Model file for the job. Use its own axes, mm. A direction names the side the tool comes from. Round coordinates to 2 decimals unless told otherwise and drop trailing zeros. Loops run counter-clockwise (first coordinate to the right, second up) from the corner with the lowest first, then second, coordinate; pieces in that order, holes last. Notation, with made-up numbers: M 9,-35 L 63,-35 A15 ccw 63,-18 Z; hole C 34.25,53.25 d10. An arc over 180 degrees is marked long. Use a Markdown table: item, result. Add a question column.
Item 1: Saw through at D-D on y = 0. Write the cut outline in (x, z), then the cut area to 3 significant figures.
Item 2: Saw through at B-B on x = -11. Write the cut outline in (y, z).
Item 3: Saw through at C-C on z = -5. Write the cut outline in (x, y) (3 decimals).
Item 4: Two-plate mould, pull along X, no slides. Class faces 1 (the cylindrical face through (15.5, -0.11, 4.88)), 2 (the cylindrical face through (-1.73, 0.04, 7.81)), 3 (the flat face through (13, 8, 8)): +X half, -X half, draft (parallel to the pull), parting line (faces both ways), or undercut.
Item 5: Pin check, flat tips, straight feed: P1, Ø2, axis at x = -6.5, y = -4.5, coming from the +Z side; P2, Ø17, axis at x = -7, z = 0, coming from the +Y side; P3, Ø1, axis at x = -8.5, y = 2, coming from the -Z side; P4, Ø2, axis at x = -3.5, z = 8.5, coming from the +Y side. Stop position of each tip, or through.
Item 6: Saw through at A-A on z = 0. Give the number of separate pieces and of enclosed holes in the cut face, then the cut area to 3 significant figures.
Item 7: Tool access for faces 4 (the flat face through (13, 7.5, -10)), 5 (the flat face through (-6, 2.5, -6)), 6 (the cylindrical face through (16.453, -7.753, 5.181)), 7 (the flat face through (6, -2.5, -6)), 8 (the flat face through (-13, -8, 8)): list every direction of +Z, -Z, +X, -X, +Y, -Y with a clear straight run to the whole face (end or side of a thin tool).
Item 8: Wall check: L1, parallel to Y at x = 15.5, z = 7.5; L2, parallel to Z at x = -5.5, y = -1.15; L3, parallel to Z at x = 0, y = -5.9. Give the ranges that are in metal, low to high. Write a range as from..to.
```python
from build123d import *

# Parameters (mm, degrees)
SKETCH2_R          = 1.25
SKETCH2_R_2        = 8
CUT_EXTRUDE1_DEPTH = 10


with BuildPart() as part:
    # Sketch1 → Revolve1 (revolve)
    with BuildSketch(Plane.XY):
        Polygon((15, 8), (17.25, 8), (17.25, 7.5), (16.25, 7.5), (16.25, -7.5), (17.25, -7.5), (17.25, -8), (15, -8), (15, -2.5), (0, -2.5), (0, 2.5), (15, 2.5), align=None)
    revolve(axis=Axis((0, 8.982990787, 0), (0, -1, 0)))

    # Sketch2 → Cut-Extrude1 (cut, symmetric)
    with BuildSketch(Plane(origin=(0, 2.5, 0), x_dir=(1, 0, 0), z_dir=(0, 1, 0))):
        with Locations((11, 0)):
            Circle(SKETCH2_R)
        with Locations((5.5, -9.526279442)):
            Circle(SKETCH2_R)
        with Locations((-5.5, -9.526279442)):
            Circle(SKETCH2_R)
        with Locations((-11, 0)):
            Circle(SKETCH2_R)
        with Locations((-5.5, 9.526279442)):
            Circle(SKETCH2_R)
        with Locations((5.5, 9.526279442)):
            Circle(SKETCH2_R)
        Circle(SKETCH2_R_2)
    extrude(amount=CUT_EXTRUDE1_DEPTH, both=True, mode=Mode.SUBTRACT)


solid = part.part
```
Entries:
| question | item | result |
|---|---|---|
| 1 | outline | C 0,0 d32.5; hole C -11,0 d2.5; hole C 0,0 d16; hole C -5.5,-9.53 d2.5; hole C -5.5,9.53 d2.5; hole C 5.5,-9.53 d2.5; hole C 5.5,9.53 d2.5; hole C 11,0 d2.5 |
| 1 | area | 599 mm2 |
| 2 | outline | M -8,-13.29 L -7.5,-13.29 L -7.5,-11.96 L 7.5,-11.96 L 7.5,-13.29 L 8,-13.29 L 8,-10.2 L 2.5,-10.2 L 2.5,-1.25 L -2.5,-1.25 L -2.5,-10.2 L -8,-10.2 Z; M -8,10.2 L -2.5,10.2 L -2.5,1.25 L 2.5,1.25 L 2.5,10.2 L 8,10.2 L 8,13.29 L 7.5,13.29 L 7.5,11.96 L -7.5,11.96 L -7.5,13.29 L -8,13.29 Z |
| 3 | outline | M -16.509,-8 L -14.142,-8 L -14.142,-2.5 L -6.245,-2.5 L -6.245,2.5 L -14.142,2.5 L -14.142,8 L -16.509,8 L -16.509,7.5 L -15.462,7.5 L -15.462,-7.5 L -16.509,-7.5 Z; M 6.245,-2.5 L 14.142,-2.5 L 14.142,-8 L 16.509,-8 L 16.509,-7.5 L 15.462,-7.5 L 15.462,7.5 L 16.509,7.5 L 16.509,8 L 14.142,8 L 14.142,2.5 L 6.245,2.5 Z |
| 4 | face 1 | parting line |
| 4 | face 2 | undercut |
| 4 | face 3 | draft |
| 5 | P1 | z = 15.29 |
| 5 | P2 | y = 8 |
| 5 | P3 | z = -14.14 |
| 5 | P4 | y = 2.5 |
| 6 | separate pieces | 4 |
| 6 | enclosed holes | 0 |
| 6 | area | 87.0 mm2 |
| 7 | face 4 | none |
| 7 | face 5 | +Y |
| 7 | face 6 | +Y, -Y |
| 7 | face 7 | -Y |
| 7 | face 8 | +Z, -Z, +X, -X, -Y |
| 8 | L1 | -8..-7.5, 7.5..8 |
| 8 | L2 | -15.29..-10.78, -8.28..-5.81, 5.81..8.28, 10.78..15.29 |
| 8 | L3 | -16.25..-15, 15..16.25 |
